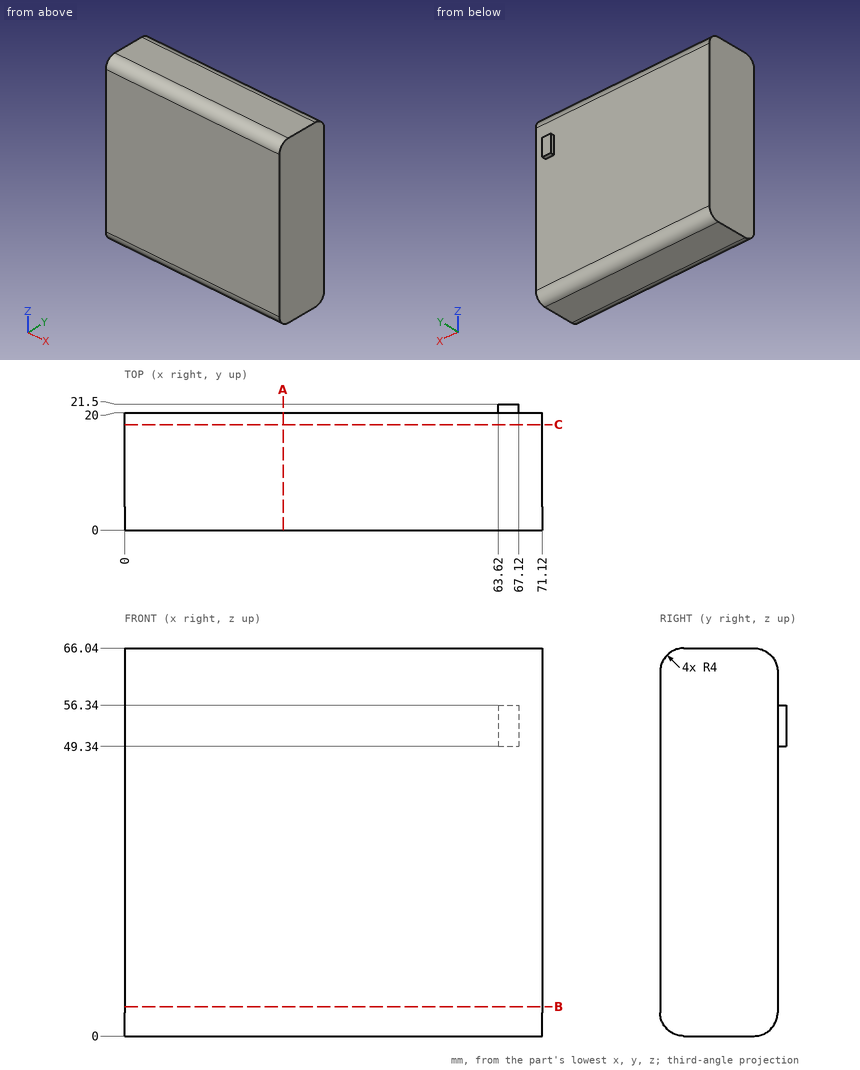
Print and shaded views of the part. All mm, measured from the part's lowest x, y and z. Round coordinates to 2 decimals unless told otherwise and drop trailing zeros. Write each loop counter-clockwise with the first axis right and the second up, starting at its lowest first coordinate (ties: lowest second). Pieces come first, ordered by that corner, then holes. Notation, with made-up numbers: (19.25, 17.25) -> (48.25, 17.25) arc R14 cw to (48.25, 39.25) -> close; hole circle Ø10 at (-22, -17.5). An arc over 180 degrees is marked (long way). Answer in a Markdown table with one row per item. Add a question column.
Item 1: Saw through at C-C, the plane y = 18. Write the cut outline in (x, z), then the cut area to 3 significant figures.
Item 2: Saw through at A-A, the plane x = 27. Write the cut outline in (y, z), then the cut area to 3 significant figures.
Item 3: Drill centre lines: line 1 (Y direction, x = 68, z = 32); line 2 (Z direction, x = 46.5, y = 19); line 3 (Z direction, x = 47.5, y = 1.5). Where is each one in solid material? Low to high. Write a range as from..to.
Item 4: Drop a flat-ended pin along its axis: pin 1 Ø1.5 at (x, z) = (34, 20) entering from +Y. Give the stop position or say it passes through.
Item 5: Saw through at B-B, the plane z = 5. Write the cut outline in (x, y).
Findings below:
| question | item | result |
|---|---|---|
| 1 | outline | (0, 0.54) -> (71.12, 0.54) -> (71.12, 65.5) -> (0, 65.5) -> close |
| 1 | area | 4,620 mm^2 |
| 2 | outline | (0, 4) arc R4 ccw to (4, 0) -> (16, 0) arc R4 ccw to (20, 4) -> (20, 62.04) arc R4 ccw to (16, 66.04) -> (4, 66.04) arc R4 ccw to (0, 62.04) -> close |
| 2 | area | 1,310 mm^2 |
| 3 | line 1 | y = 0..20 |
| 3 | line 2 | z = 1.35..64.69 |
| 3 | line 3 | z = 0.88..65.16 |
| 4 | pin 1 | stops at y = 20 |
| 5 | outline | (0, 0) -> (71.12, 0) -> (71.12, 20) -> (0, 20) -> close |
